The drawing under review shows one solid part. Ordinate dimensions are in mm from its lowest x, y, z. Give positions to 0.01 mm unless a question says otherwise; leave off trailing zeros. Order: outer loops, then holes, each group sorted by start corner. A loop starts at its lowest first (then second) coordinate and runs counter-clockwise, first axis right, second up. Notation, with made-up numbers: (-18.5, 12.25) - (33.5, 12.25) arc R31 ccw to (33.5, 47.25) - close; hole circle Ø11 at (-35.75, -30.5). An arc over 180 degrees is marked (long way). Write item = value, one per line. Start each with the question number.
1. Mouldability with a two-part tool opening along X and no side actions: class the marked faces 1 and 2 as pulls with the +X half, pulls with the -X half, needs draft (parallel to the pull), parting line crosses it, or undercut.
2. For P1, Ø3, axis at x = 24.9, y = 6.325, coming from the +Z side, flat-tipped, find the tip position at first contact; note if it passes through.
3. We need section A-A, the plane y = 20.5. Give the boundary of the cut face in (x, z).
4. Wall thickness on probe 1 along X at (y, z) = (17, 0.9); probe 2 along X at (y, z) = (24.9, 1.65) (3 decimals): over which ranges is each line inside the solid? List them lowest first.
5. We need section C-C, the plane z = 0.6. State how many separate pieces and enclosed holes the cut face has, and give its area (3 significant figures).
6. We need section B-B, the plane x = 16.1. Give the boundary of the cut face in (y, z) (3 decimals), and give its area (3 significant figures).
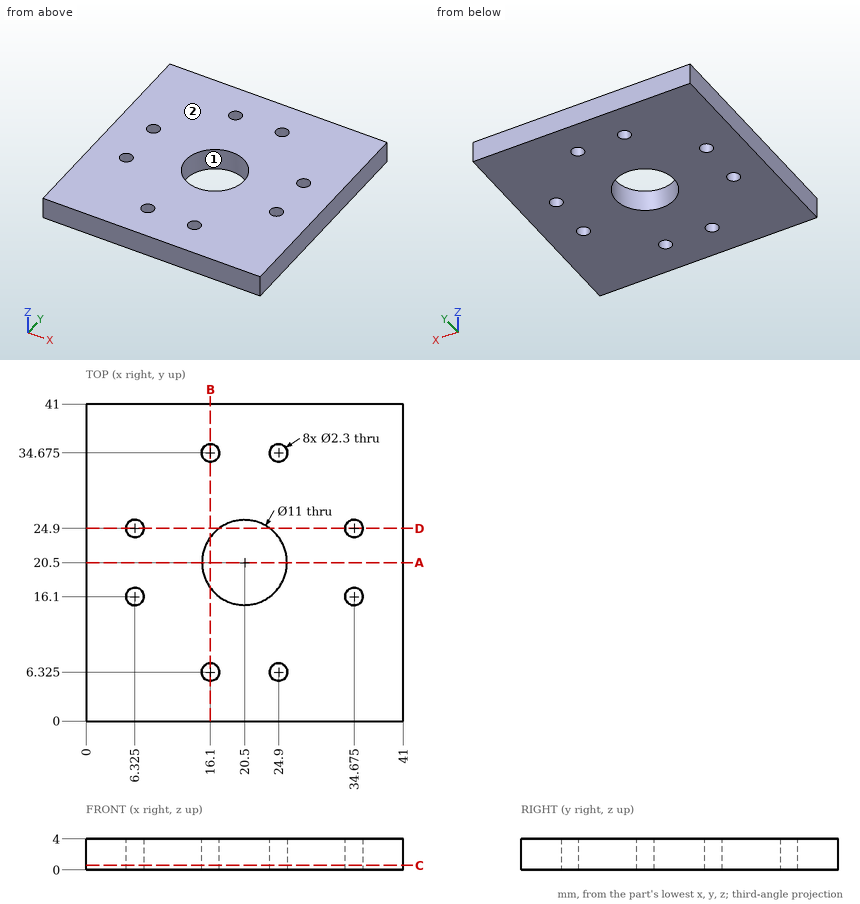
Model answer:
q1.face_1 = undercut
q1.face_2 = needs draft
q2.P1 = 4
q3.outline = (0, 0) - (15, 0) - (15, 4) - (0, 4) - close; (26, 0) - (41, 0) - (41, 4) - (26, 4) - close
q4.probe_1 = 0 to 5.61, 7.04 to 16.26, 24.74 to 33.96, 35.39 to 41
q4.probe_2 = 0 to 5.175, 7.475 to 17.2, 23.8 to 33.525, 35.825 to 41
q5.separate_pieces = 1
q5.enclosed_holes = 9
q5.area = 1,550 mm2
q6.outline = (0, 0) - (5.175, 0) - (5.175, 4) - (0, 4) - close; (7.475, 0) - (17.2, 0) - (17.2, 4) - (7.475, 4) - close; (23.8, 0) - (33.525, 0) - (33.525, 4) - (23.8, 4) - close; (35.825, 0) - (41, 0) - (41, 4) - (35.825, 4) - close
q6.area = 119 mm2
